The model under review builds one solid part; all positions refer to its coordinate system, in mm. Face numbers are marked on the shaded views. Give positions to 0.01 mm unless a question says otherwise; leave off trailing zeros. Order: outer loops, then holes, each group sorted by start corner. A loop starts at its lowest first (then second) coordinate and runs counter-clockwise, first axis right, second up. Notation, with made-up numbers: (75, -22.5) - (87, -22.5) arc R16 cw to (87, -0.5) - close; hole circle Ø10 at (46.5, -19). An arc over 180 degrees is marked (long way). Use a Markdown table: item, result. Add a question column.
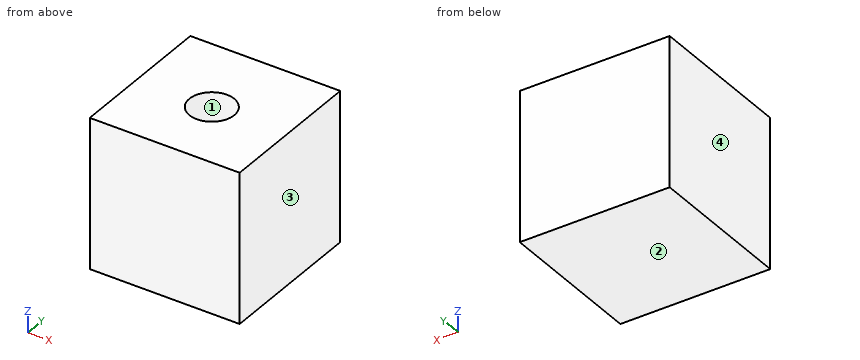
```python
from build123d import *

# Parameters (mm, degrees)
F0_W     = 150
F0_H     = 150
F1_DEPTH = 150
F3_D     = 45
F3_DEPTH = 58
F3_TIP   = 13.5193639281


with BuildPart() as f1:
    # F0 (on Front) → F1 (new body)
    with BuildSketch(Plane.XZ):
        Rectangle(F0_W, F0_H)
    extrude(amount=F1_DEPTH)

    # F3
    with Locations(Plane.XY.offset(75)):
        with Locations((0, -79.7429457307)):
            Hole(F3_D / 2, depth=F3_DEPTH)
            with Locations((0, 0, -(F3_DEPTH + F3_TIP / 2))):  # 118° drill point
                Cone(0, F3_D / 2, F3_TIP, mode=Mode.SUBTRACT)


solid = f1.part
```
Q1. Wall thickness on probe 1 along Y at (x, z) = (0, 29); probe 2 along X at (y, z) = (-90, 38.5); probe 3 along Z at (x, y) = (14.5, -96): over which ranges is each line inside the solid? List them lowest first.
Q2. We need section A-A (z = 20). Write out the cut boundary in (x, y), plus the area to 3 significant figures.
Q3. Draft analysis for pull direction X (two halves, no side actions). For the marked faces 1, 2, 3 and 4, state which applies: pulls with the +X half, pulls with the -X half, needs draft (parallel to the pull), parting line crosses it, or undercut.
Here are the results:
| question | item | result |
|---|---|---|
| 1 | probe 1 | -150 to -102.24, -57.24 to 0 |
| 1 | probe 2 | -75 to -20.03, 20.03 to 75 |
| 1 | probe 3 | -75 to 16.57 |
| 2 | outline | (-75, -150) - (75, -150) - (75, 0) - (-75, 0) - close; hole circle Ø45 at (0, -79.74) |
| 2 | area | 20,900 mm2 |
| 3 | face 1 | undercut |
| 3 | face 2 | needs draft |
| 3 | face 3 | pulls with the +X half |
| 3 | face 4 | pulls with the -X half |
